Geometry check sheet. Reference: the model listing, model coordinates, mm. Round coordinates to 2 decimals unless told otherwise and drop trailing zeros. Write each loop counter-clockwise with the first axis right and the second up, starting at its lowest first coordinate (ties: lowest second). Pieces come first, ordered by that corner, then holes. Notation, with made-up numbers: (10.25, 30.5) - (63.25, 30.5) arc R18 cw to (63.25, 38.5) - close; hole circle Ø3 at (22, -17.75). An arc over 180 degrees is marked (long way). Return JSON: item names as keys, results as strings.
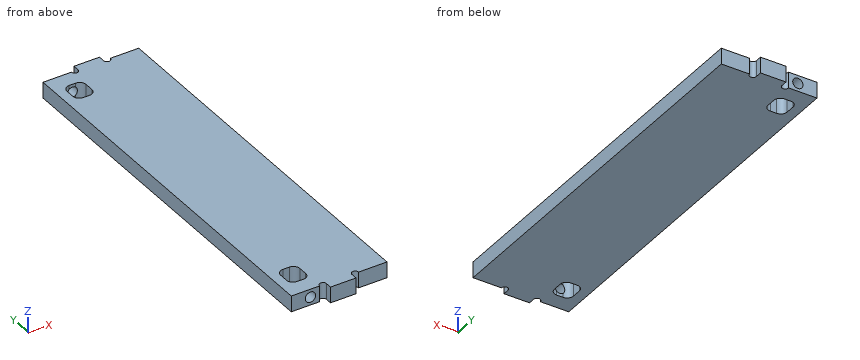
Autodesk Inventor part; units mm, degrees
ref_plane "YZ Plane" through (0, 0, 0) normal (1, 0, 0) x (0, 1, 0)
ref_plane "XZ Plane" through (0, 0, 0) normal (0, 1, 0) x (-1, 0, 0)
ref_plane "XY Plane" through (0, 0, 0) normal (0, 0, 1) x (1, 0, 0)
sketch "スケッチ1" plane through (0, 0, 0) normal (0, 0, 1) x (1, 0, 0)
  line L0 (15, 60.5) -> (-15, 60.5) construction
  line L1 (-15, 60.5) -> (-15, -60.5)
  line L2 (-15, -60.5) -> (15, -60.5)
  line L3 (15, -60.5) -> (15, 60.5)
  line L4 (15, 60.5) -> (-15, -60.5) construction
  line L5 (-15, 60.5) -> (15, -60.5) construction
  line L6 (4, 60.5) -> (4, 62.5)
  line L7 (4, 62.5) -> (-4, 62.5)
  arc A0 (4, 60.5) -> (6.1, 60.5) centre (5.05, 60.5) ccw
  line L8 (0, 62.5) -> (0, 60.5) construction
  line L9 (-4, 60.5) -> (-4, 62.5)
  arc A1 (-6.1, 60.5) -> (-4, 60.5) centre (-5.05, 60.5) ccw
  line L10 (0, 60.5) -> (0, -60.5) construction
  line L11 (15, 0) -> (-15, 0)
  line L12 (-9, 60.5) -> (-9, 55.5) construction
  line L13 (-11, 60.5) -> (-11, 55.5) construction
  line L14 (-7, 60.5) -> (-7, 55.5) construction
  line L15 (11.6254, -55.5) -> (-12, -55.5) construction
  line L16 (-12, -55.5) -> (-12, 55.5) construction
  line L17 (-12, 55.5) -> (11.6254, 55.5) construction
  line L18 (11.6254, 55.5) -> (11.6254, -55.5) construction
  line L19 (11.6254, -55.5) -> (-12, 55.5) construction
  line L20 (-12, -55.5) -> (11.6254, 55.5) construction
  line L21 (-8, 55.5) -> (-10, 55.5)
  line L22 (-12, 53.5) -> (-12, 50.6397)
  line L23 (-10, 48.6397) -> (-8, 48.6397)
  line L24 (-6, 50.6397) -> (-6, 53.5)
  line L25 (-6, 55.5) -> (-12, 48.6397) construction
  line L26 (-12, 55.5) -> (-6, 48.6397) construction
  arc A2 (-6, 53.5) -> (-8, 55.5) centre (-8, 53.5) ccw
  arc A3 (-10, 55.5) -> (-12, 53.5) centre (-10, 53.5) ccw
  arc A4 (-12, 50.6397) -> (-10, 48.6397) centre (-10, 50.6397) ccw
  arc A5 (-8, 48.6397) -> (-6, 50.6397) centre (-8, 50.6397) ccw
  line L27 (6.1, 60.5) -> (15, 60.5)
  line L28 (-6.1, 60.5) -> (-15, 60.5)
  point P0 (0, 0)
  point P1 (-0.1873, 0)
  point P2 (-9, 52.0698)
  point P3 (-9, 52.0698)
  dimension "d0" = 30
  dimension "d1" = 121
  dimension "d2" = 1.05
  dimension "d3" = 2
  dimension "d4" = 0
  dimension "d5" = 8
  dimension "d6" = 5
  dimension "d7" = 3
  dimension "d8" = 4
  dimension "d9" = 9
  dimension "d10" = 2
extrude "押し出し1" add sketch "スケッチ1" along normal blind 5 contours L28 A1 L9 L7 L6 A0 L27 L3 L11 L1
sketch "スケッチ2" plane through (-15, 60.5, 0) normal (0, 1, 0) x (1, 0, 0)
  line L0 (0, 0) -> (0, -5)
  line L1 (0, -2.5) -> (30, -2.5)
  line L2 (30, 0) -> (30, -5)
  line L3 (15, 0) -> (15, -5)
  line L4 (19, -5) -> (11, -5)
  point P0 (6, -2.5)
  dimension "d13" = 9
hole "穴1" at (-9, 60.5, 2.5) direction (0, -1, 0) diameter 3.242 depth 5 tip angle 118
mirror "ミラー1" about plane through (-15, 0, 0) normal (0, -1, 0)
properties part number "Trunk_back_waisit_frame_" material "アセタール樹脂、黒"
(1) Section check A-A, the plane x = 5.05. Enter the section's corners in (y, z), plus the area to 4 significant figures.
Response values:
{"outline": "(-59.45, 0) - (59.45, 0) - (59.45, 5) - (-59.45, 5) - close", "area": "594.5 mm^2"}
(2) Section check B-B, the plane x = 10.25. Enter the section's corners in (y, z).
Response values:
{"outline": "(-60.5, 0) - (60.5, 0) - (60.5, 5) - (-60.5, 5) - close"}
(3) Gauge pin test, flat ends, axial feed: pin 1 (2.5 mm diameter, centred on x = 11, z = 3.5, fed in from +Y); pin 2 (0.6 mm diameter, centred on x = -9, z = 1.5, fed in from -Y); pin 3 (2.5 mm diameter, centred on x = -9, z = 2.5, fed in from -Y). Record the tip position at first contact, or that the pin passes through.
Response values:
{"pin 1": "stops at y = 60.5", "pin 2": "stops at y = -48.64", "pin 3": "stops at y = -48.66"}
(4) Material ranges on line 1 along X through (y, z) = (58.55, 2.5); line 2 along Z through (x, y) = (-9, 56.7); line 3 along Y through (x, z) = (-10, 1.55), recorded low to high. Write a range as [from, to].
Response values:
{"line 1": "x = [-15, -10.62], [-7.38, 15]", "line 2": "z = [0, 0.88], [4.12, 5]", "line 3": "y = [-48.64, 48.64]"}
